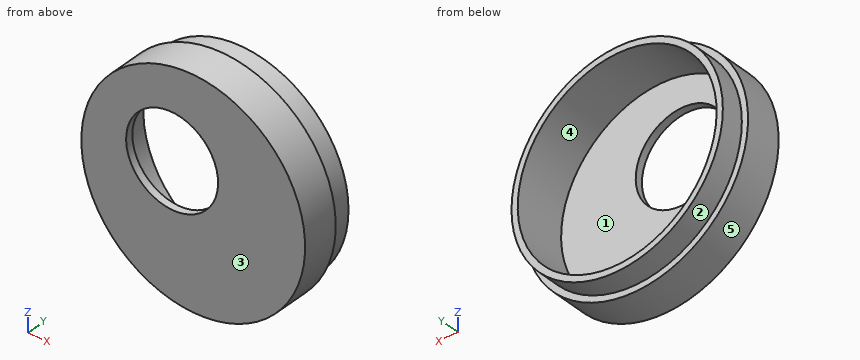
```python
from build123d import *

# Parameters (mm, degrees)
CUT_EXTRUDE1_REACH  = 36.551
SKETCH2_R           = 22.225
SKETCH2_R_2         = 21.59
SKETCH3_R           = 9.398
CUT_EXTRUDE2_DEPTH  = 35.551469781
SKETCH5_R           = 20.955
SKETCH5_R_2         = 20.32
BOSS_EXTRUDE1_DEPTH = 10.668


with BuildPart() as part:
    # Sketch1 → Revolve1 (revolve)
    with BuildSketch(Plane.XY, mode=Mode.PRIVATE) as revolve1_sk:
        Polygon((22.86, 0), (22.86, -7.52475), (0, -7.52475), (0, -6.00075), (20.955, -6.00075), (20.955, 4.66725), (22.225, 4.66725), (22.225, 2.286), (21.59, 2.286), (21.59, 0), (22.225, 0), align=None)
    revolve(revolve1_sk.sketch.rotate(Axis((0, 33.267670174, 0), (0, -1, 0)), 90), axis=Axis((0, 33.267670174, 0), (0, -1, 0)))

    # Sketch2 → Cut-Extrude1 (cut, up to next)
    with BuildSketch(Plane(origin=(0, 4.66725, 0), x_dir=(1, 0, 0), z_dir=(0, 1, 0)), mode=Mode.PRIVATE) as cut_extrude1_sk1:
        Circle(SKETCH2_R)
        with Locations(Location((0, 0, 0), (0, 0, 270))):
            Circle(SKETCH2_R_2, mode=Mode.SUBTRACT)
    cut_extrude1_tool1 = extrude(cut_extrude1_sk1.sketch, amount=-CUT_EXTRUDE1_REACH, mode=Mode.PRIVATE) & part.part
    add(cut_extrude1_tool1.solids().sort_by_distance((-21.596382, 4.66725, 0))[0], mode=Mode.SUBTRACT)

    # Sketch3 → Cut-Extrude2 (cut, through all)
    with BuildSketch(Plane.XZ.offset(7.52475)):
        with Locations(Location((-4.318, 4.318, 0), (0, 0, 270))):
            Circle(SKETCH3_R)
    extrude(amount=-CUT_EXTRUDE2_DEPTH, mode=Mode.SUBTRACT)

    # Sketch5 → Boss-Extrude1 (add)
    with BuildSketch(Plane(origin=(0, 4.66725, 0), x_dir=(1, 0, 0), z_dir=(0, 1, 0))):
        Circle(SKETCH5_R)
        with Locations(Location((0, 0, 0), (0, 0, 270))):
            Circle(SKETCH5_R_2, mode=Mode.SUBTRACT)
    extrude(amount=-BOSS_EXTRUDE1_DEPTH)


solid = part.part
```
Can you work these out from the model? Positions are in its coordinate system, mm. Face numbers are marked on the shaded views. A direction names the side the tool comes from. Give positions to 0.01 mm unless a question says otherwise; leave off trailing zeros. Loops run counter-clockwise (first coordinate to the right, second up) from the corner with the lowest first, then second, coordinate; pieces in that order, holes last. Notation, with made-up numbers: M 24.5,-8.75 L 69.5,-8.75 A33 ccw 69.5,27.25 Z; hole C 43.5,69 d7. An arc over 180 degrees is marked long. Use CSV: the item, a comma, the result in double quotes. Start each with the question number.
1. Imagine slicing it at A-A, the plane x = -5. Write out the boundary of the cut face in (y, z), plus the area to 3 significant figures.
2. On a 3-axis mill with a long thin cutter (end or side, diameter ignored), from which of +Z, -Z, +X, -X, +Y, -Y can I reach the whole of each face in a straight line? I mean the marked faces 4 and 5. Say none if no direction works.
3. Imagine slicing it at D-D, the plane z = 18. Write out the boundary of the cut face in (x, y).
4. If we mould it in two halves opening along X, with no side actions, what happens to the marked faces 1, 2 and 3? For each: released by +X, released by -X, zero draft, split by the parting line, or undercut.
5. If I drill on L1, parallel to X at y = -0.5, z = 0; L2, parallel to Y at x = -12, z = -10.5; L3, parallel to Z at x = -3, y = -4, over which ranges is the centre line in solid material (lowest first)?
6. For P1, Ø4, axis at y = -2.5, z = -11, coming from the -X side; P2, Ø1, axis at x = -13, z = -1, coming from the +Y side; P3, Ø6, axis at y = 2.5, z = 6, coming from the -X side, each with a flat end and sliding along its axis, tell me the tip position at first contact or that it passes through.
7. Imagine slicing it at B-B, the plane z = 7. Write out the boundary of the cut face in (x, y), plus the area to 3 significant figures.
8. Imagine slicing it at C-C, the plane y = 3.75. Write out the boundary of the cut face in (x, z).
Response values:
1,outline,"M -7.52,-22.31 L 0,-22.31 L 0,-21 L 4.67,-21 L 4.67,-19.7 L -6,-19.7 L -6,-5.06 L -7.52,-5.06 Z; M -7.52,13.69 L -6,13.69 L -6,19.7 L 4.67,19.7 L 4.67,21 L 0,21 L 0,22.31 L -7.52,22.31 Z"
1,area,"83.0 mm^2"
2,face 4,"+Y"
2,face 5,"+Y, -Y"
3,outline,"M -14.09,-7.52 L 14.09,-7.52 L 14.09,0 L 11.92,0 L 11.92,4.67 L 9.43,4.67 L 9.43,-6 L -9.43,-6 L -9.43,4.67 L -11.92,4.67 L -11.92,0 L -14.09,0 Z"
4,face 1,"undercut"
4,face 2,"split by the parting line"
4,face 3,"zero draft"
5,L1,"-22.86 to -20.32, 20.32 to 22.86"
5,L2,"-7.52 to -6"
5,L3,"-22.66 to -20.1, 20.1 to 22.66"
6,P1,"x = -21.01"
6,P2,"y = -6"
6,P3,"x = -22.44"
7,outline,"M -21.76,-7.52 L -13.33,-7.52 L -13.33,-6 L -19.08,-6 L -19.08,4.67 L -20.42,4.67 L -20.42,0 L -21.76,0 Z; M 4.69,-7.52 L 21.76,-7.52 L 21.76,0 L 20.42,0 L 20.42,4.67 L 19.08,4.67 L 19.08,-6 L 4.69,-6 Z"
7,area,"83.7 mm^2"
8,outline,"C 0,0 d43.18; hole C 0,0 d40.64"
